Check sheet for the modelled part. Datum: model origin and axes. Units: mm. A direction names the side the tool comes from. Round coordinates to 2 decimals unless told otherwise and drop trailing zeros. Order: outer loops, then holes, each group sorted by start corner. A loop starts at its lowest first (then second) coordinate and runs counter-clockwise, first axis right, second up. Notation, with made-up numbers: (23, -12) -> (35, -12) arc R23 ccw to (35, 1) -> close; hole circle Ø1 at (-4.75, -31.75). An arc over 180 degrees is marked (long way). Answer in a Markdown table with one row per item.
from build123d import *

# Parameters (mm, degrees)
SKETCH1_W               = 50.8
SKETCH1_H               = 50.8
BOSS_EXTRUDE1_DEPTH     = 69.85
SHELL1_T                = -3.175
SKETCH2_W               = 31.75
SKETCH2_H               = 26.9875
CUT_EXTRUDE1_DEPTH      = 79.545162168
FILLET1_R               = 3.175
CUT_EXTRUDE2_DEPTH      = 79.545162168
CUT_EXTRUDE2_DEPTH_BACK = 79.545162168
SKETCH3_R               = 3.175
CUT_EXTRUDE3_DEPTH      = 79.545162168
CUT_EXTRUDE3_DEPTH_BACK = 79.545162168
SKETCH4_R               = 2.4892
CUT_EXTRUDE4_DEPTH      = 79.545162168
CUT_EXTRUDE4_DEPTH_BACK = 79.545162168
SKETCH5_R               = 2.4892
FILLET2_R               = 3.175


with BuildPart() as part:
    # Sketch1 → Boss-Extrude1 (new, symmetric)
    with BuildSketch(Plane.XY):
        Rectangle(SKETCH1_W, SKETCH1_H)
    extrude(amount=BOSS_EXTRUDE1_DEPTH, both=True)

    # Shell1
    shell1_openings = [part.faces().sort_by_distance(p)[0] for p in [
        (0, 0, 69.85),
        (0, 0, -69.85),
    ]]
    offset(amount=SHELL1_T, openings=shell1_openings, kind=Kind.INTERSECTION)

    # Sketch2 → Cut-Extrude1 (cut, through all)
    with BuildSketch(Plane(origin=(0, 0, 0), x_dir=(1, 0, 0), z_dir=(0, 1, 0))):
        with Locations((0, 31.75)):
            Rectangle(SKETCH2_W, SKETCH2_H)
        with Locations((0, -47.625)):
            Rectangle(SKETCH2_W, SKETCH2_H)
    extrude(amount=CUT_EXTRUDE1_DEPTH, mode=Mode.SUBTRACT)

    # Fillet1
    fillet1_edges = [part.edges().sort_by_distance(p)[0] for p in [
        (15.875, 23.8125, -18.25625),
        (15.875, 23.8125, -45.24375),
        (-15.875, 23.8125, -45.24375),
        (-15.875, 23.8125, -18.25625),
    ]]
    fillet(fillet1_edges, radius=FILLET1_R)

    # Sketch3 → Cut-Extrude2 (cut, two sides: drawn at the far end of the back side and taken through both)
    with BuildSketch(Plane(origin=(0, 0, 0), x_dir=(0, 0, -1), z_dir=(1, 0, 0)).offset(-CUT_EXTRUDE2_DEPTH_BACK)):
        with Locations((31.75, 9.525)):
            Circle(SKETCH3_R)
        with Locations((-44.45, 9.525)):
            Circle(SKETCH3_R)
    extrude(amount=CUT_EXTRUDE2_DEPTH + CUT_EXTRUDE2_DEPTH_BACK, mode=Mode.SUBTRACT)

    # Sketch4 → Cut-Extrude3 (cut, two sides: drawn at the far end of the back side and taken through both)
    with BuildSketch(Plane(origin=(0, 0, 0), x_dir=(0, 0, -1), z_dir=(1, 0, 0)).offset(-CUT_EXTRUDE3_DEPTH_BACK)):
        with Locations((57.15, 12.7)):
            Circle(SKETCH4_R)
        with Locations((44.45, -12.7)):
            Circle(SKETCH4_R)
        with Locations((31.75, -12.7)):
            Circle(SKETCH4_R)
        with Locations((19.05, -12.7)):
            Circle(SKETCH4_R)
        with Locations((57.15, 0)):
            Circle(SKETCH4_R)
        with Locations((57.15, -12.7)):
            Circle(SKETCH4_R)
        with Locations((-61.9125, 12.7)):
            Circle(SKETCH4_R)
        with Locations((-23.8125, 12.7)):
            Circle(SKETCH4_R)
        with Locations((-11.1125, 12.7)):
            Circle(SKETCH4_R)
        with Locations((-23.8125, 0)):
            Circle(SKETCH4_R)
        with Locations((-11.1125, 0)):
            Circle(SKETCH4_R)
        with Locations((-49.2125, -12.7)):
            Circle(SKETCH4_R)
        with Locations((-36.5125, -12.7)):
            Circle(SKETCH4_R)
        with Locations((-23.8125, -12.7)):
            Circle(SKETCH4_R)
        with Locations((-11.1125, -12.7)):
            Circle(SKETCH4_R)
        with Locations((-61.9125, 0)):
            Circle(SKETCH4_R)
        with Locations((-61.9125, -12.7)):
            Circle(SKETCH4_R)
    extrude(amount=CUT_EXTRUDE3_DEPTH + CUT_EXTRUDE3_DEPTH_BACK, mode=Mode.SUBTRACT)

    # Sketch5 → Cut-Extrude4 (cut, two sides: drawn at the far end of the back side and taken through both)
    with BuildSketch(Plane(origin=(0, 0, 0), x_dir=(1, 0, 0), z_dir=(0, 1, 0)).offset(-CUT_EXTRUDE4_DEPTH_BACK)):
        with Locations(Location((-12.7, -57.15, 0), (0, 0, 270))):
            Circle(SKETCH5_R)
        with Locations(Location((0, -57.15, 0), (0, 0, 270))):
            Circle(SKETCH5_R)
        with Locations(Location((12.7, -57.15, 0), (0, 0, 270))):
            Circle(SKETCH5_R)
    extrude(amount=CUT_EXTRUDE4_DEPTH + CUT_EXTRUDE4_DEPTH_BACK, mode=Mode.SUBTRACT)

    # Fillet2
    fillet2_edges = [part.edges().sort_by_distance(p)[0] for p in [
        (15.875, 23.8125, 61.11875),
        (15.875, 23.8125, 34.13125),
        (-15.875, 23.8125, 34.13125),
        (-15.875, 23.8125, 61.11875),
    ]]
    fillet(fillet2_edges, radius=FILLET2_R)


solid = part.part
Item 1: Set-up check for faces 1 (the flat face through (15.875, 24, 48)), 2 (the cylindrical face through (23.79, 0.109, -54.663)), 3 (the flat face through (0, -22.225, 1)): record each of +Z, -Z, +X, -X, +Y, -Y from which the full face is reachable in a straight line by a thin tool's end or side.
Result sheet:
| item | result |
|---|---|
| face 1 | +Y |
| face 2 | +X, -X |
| face 3 | +Z, -Z |
Item 2: Scan lines: line 1 (Y direction, x = -23.1, z = -57.15); line 2 (Y direction, x = -16, z = 54.5) (3 decimals). Record each from-to range of solid material in increasing order. Write a range as [from, to].
Result sheet:
| item | result |
|---|---|
| line 1 | y = [-25.4, -15.19], [-10.21, -2.49], [2.49, 10.21], [15.19, 25.4] |
| line 2 | y = [-25.4, -22.225], [22.225, 25.4] |
Item 3: Cross-section at C-C (z = 29). Record the boundary of the cut face in (x, y) (3 decimals).
Result sheet:
| item | result |
|---|---|
| outline | (-25.4, -25.4) -> (25.4, -25.4) -> (25.4, 25.4) -> (-25.4, 25.4) -> close; hole (-22.225, -22.225) -> (22.225, -22.225) -> (22.225, 22.225) -> (-22.225, 22.225) -> close |
Item 4: Cross-section at D-D (z = 44.45). Record the boundary of the cut face in (x, y) (3 decimals), and give its area (3 significant figures).
Result sheet:
| item | result |
|---|---|
| outline | (-25.4, -25.4) -> (25.4, -25.4) -> (25.4, 6.35) -> (22.225, 6.35) -> (22.225, -22.225) -> (-22.225, -22.225) -> (-22.225, 6.35) -> (-25.4, 6.35) -> close; (-25.4, 12.7) -> (-22.225, 12.7) -> (-22.225, 22.225) -> (-15.875, 22.225) -> (-15.875, 25.4) -> (-25.4, 25.4) -> close; (15.875, 22.225) -> (22.225, 22.225) -> (22.225, 12.7) -> (25.4, 12.7) -> (25.4, 25.4) -> (15.875, 25.4) -> close |
| area | 464 mm^2 |
Item 5: Cross-section at A-A (x = 4.5). Record the boundary of the cut face in (y, z) (3 decimals), and give its area (3 significant figures).
Result sheet:
| item | result |
|---|---|
| outline | (-25.4, -69.85) -> (-22.225, -69.85) -> (-22.225, 69.85) -> (-25.4, 69.85) -> close; (22.225, -69.85) -> (25.4, -69.85) -> (25.4, -45.244) -> (22.225, -45.244) -> close; (22.225, -18.256) -> (25.4, -18.256) -> (25.4, 34.131) -> (22.225, 34.131) -> close; (22.225, 61.119) -> (25.4, 61.119) -> (25.4, 69.85) -> (22.225, 69.85) -> close |
| area | 716 mm^2 |
Item 6: Cross-section at B-B (z = -57.15). State how many separate pieces and enclosed holes the cut face has, and give its area (3 significant figures).
Result sheet:
| item | result |
|---|---|
| separate pieces | 6 |
| enclosed holes | 0 |
| area | 510 mm^2 |
Item 7: Mould release check, pull along Z, two halves, no side actions. Record for faces 4 (the flat face through (0, 22.225, 1)), 5 (the cylindrical face through (-14.97, 23.835, 60.164)), 6 (the flat face through (-23, 0, 69.85)): pulls with the +Z half, pulls with the -Z half, needs draft (parallel to the pull), parting line crosses it, or undercut.
Result sheet:
| item | result |
|---|---|
| face 4 | needs draft |
| face 5 | undercut |
| face 6 | pulls with the +Z half |
Item 8: Depth check by flat-ended pin: P1, Ø3, axis at y = -12.7, z = 36.51, coming from the +X side; P2, Ø5.5, axis at x = -12.7, z = 57.15, coming from the +Y side (3 decimals). Enter the tip coordinate at first touch or a pass-through.
Result sheet:
| item | result |
|---|---|
| P1 | passes through |
| P2 | stops at y = -22.225 |
